For this review, take the finished solid that the model builds, in its own axes (mm). Round coordinates to 2 decimals unless told otherwise and drop trailing zeros. Order: outer loops, then holes, each group sorted by start corner. A loop starts at its lowest first (then second) coordinate and runs counter-clockwise, first axis right, second up. Notation, with made-up numbers: (56.25, -34) -> (75.25, -34) arc R26 ccw to (75.25, 0) -> close; hole circle Ø6 at (29, -16.5). An arc over 180 degrees is marked (long way). Answer in a Markdown table with one row per item.
```python
from build123d import *

# Parameters (mm, degrees)
BOSS_EXTRUDE1_DEPTH = 19.05
CHAMFER1_SIZE       = 2.54


with BuildPart() as part:
    # Sketch1 → Boss-Extrude1 (new body)
    with BuildSketch(Plane(origin=(0, 0, 0), x_dir=(1, 0, 0), z_dir=(0, 1, 0))):
        Polygon((1211.5165, 0), (1211.5165, 669.925), (2035.429, 669.925), (2035.429, 0), (2438.4, 0), (2438.4, 1219.2), (0, 1219.2), (0, 803.275), (685.8, 803.275), (685.8, 295.275), (0, 295.275), (0, 0), align=None)
    extrude(amount=-BOSS_EXTRUDE1_DEPTH)

    # Chamfer1
    chamfer1_edges = [part.edges().sort_by_distance(p)[0] for p in [
        (0, 0, -147.6375),
        (342.9, 0, -295.275),
        (685.8, 0, -549.275),
        (342.9, 0, -803.275),
        (0, 0, -1011.2375),
        (1219.2, 0, -1219.2),
        (2438.4, 0, -609.6),
        (2236.9145, 0, 0),
        (2035.429, 0, -334.9625),
        (1623.47275, 0, -669.925),
        (1211.5165, 0, -334.9625),
        (605.75825, 0, 0),
    ]]
    chamfer(chamfer1_edges, length=CHAMFER1_SIZE)


solid = part.part
```
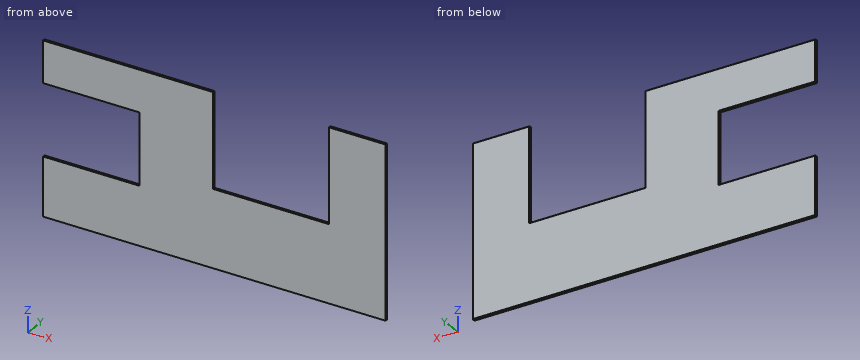
Q1. Take a section at C-C, the plane z = -180.5. Write out the cut boundary in (x, y), then the cut area to 3 significant figures.
Answer key:
| item | result |
|---|---|
| outline | (0, -19.05) -> (1211.52, -19.05) -> (1211.52, -2.54) -> (1208.98, 0) -> (2.54, 0) -> (0, -2.54) -> close; (2035.43, -19.05) -> (2438.4, -19.05) -> (2438.4, -2.54) -> (2435.86, 0) -> (2037.97, 0) -> (2035.43, -2.54) -> close |
| area | 30,700 mm^2 |
Q2. Take a section at A-A, the plane z = -324. Write out the cut boundary in (x, y).
Answer key:
| item | result |
|---|---|
| outline | (685.8, -19.05) -> (1211.52, -19.05) -> (1211.52, -2.54) -> (1208.98, 0) -> (688.34, 0) -> (685.8, -2.54) -> close; (2035.43, -19.05) -> (2438.4, -19.05) -> (2438.4, -2.54) -> (2435.86, 0) -> (2037.97, 0) -> (2035.43, -2.54) -> close |
Q3. Clearance check with flat-ended pins moving along their axes: pin 1 Ø5 at (x, y) = (497, -12.5) entering from +Z; pin 2 Ø3 at (x, y) = (1992, -2.5) entering from +Z (3 decimals); pin 3 Ø5 at (y, z) = (-13, -305) entering from -X. State where each tip first meets the part, or that it passes through.
Answer key:
| item | result |
|---|---|
| pin 1 | stops at z = 0 |
| pin 2 | stops at z = -669.925 |
| pin 3 | stops at x = 685.8 |
Q4. To check wall thickness, follow probe 1 along X at (y, z) = (-2.5, -246); probe 2 along Z at (x, y) = (355, -14) (3 decimals); probe 3 along X at (y, z) = (-3, -126.5). State the ranges of each line that lie inside material, in increasing order.
Answer key:
| item | result |
|---|---|
| probe 1 | x = 0.04 to 1211.48, 2035.47 to 2438.36 |
| probe 2 | z = -1219.2 to -803.275, -295.275 to 0 |
| probe 3 | x = 0 to 1211.52, 2035.43 to 2438.4 |
Q5. Take a section at B-B, the plane y = -11.75. Write out the cut boundary in (x, z) (1 decimal).
Answer key:
| item | result |
|---|---|
| outline | (0, -1219.2) -> (2438.4, -1219.2) -> (2438.4, 0) -> (2035.4, 0) -> (2035.4, -669.9) -> (1211.5, -669.9) -> (1211.5, 0) -> (0, 0) -> (0, -295.3) -> (685.8, -295.3) -> (685.8, -803.3) -> (0, -803.3) -> close |
Q6. Take a section at D-D, the plane x = 1635. Write out the cut boundary in (y, z) (3 decimals), then the cut area to 3 significant figures.
Answer key:
| item | result |
|---|---|
| outline | (-19.05, -1219.2) -> (-2.54, -1219.2) -> (0, -1216.66) -> (0, -672.465) -> (-2.54, -669.925) -> (-19.05, -669.925) -> close |
| area | 10,500 mm^2 |
